CAD build for the part. Positions are in the model's coordinates, mm. A direction names the side the tool comes from. Coordinates: 2 decimals unless noted, no trailing zeros. Order: outer loops, then holes, each group sorted by start corner. A loop starts at its lowest first (then second) coordinate and runs counter-clockwise, first axis right, second up. Notation, with made-up numbers: (5, 16.5) - (41, 16.5) arc R18 ccw to (41, 28.5) - close; hole circle Ø3 at (-21, -3). An arc over 180 degrees is marked (long way). Write each question's results on one line, items separated by ' | '. Start each with the question number.
Q1. Wall check: probe 1 along X at (y, z) = (30.2, 5); probe 2 along Y at (x, z) = (-11, 13.5); probe 3 along Z at (x, y) = (-20.5, 35). Give the ranges that are in metal, low to high.
Q2. Pin check, flat tips, straight feed: P1, Ø4, axis at x = 12, y = 19.5, coming from the -Z side; P2, Ø3, axis at x = -13.75, z = 5, coming from the -Y side; P3, Ø1.5, axis at y = 20, z = -35, coming from the +X side. Stop position of each tip, or through.
Q3. Band-saw the part on C-C, the plane y = 16.5. Write the cut outline in (x, z), then the cut area to 3 significant figures.
Q4. Which spindle directions (+Z, -Z, +X, -X, +Y, -Y) get a long thin tool onto all of the face, cutting with end or side? Do faces 1 (the flat face through (-27, 31.4, -1)), 2 (the flat face through (-27, 29.4, -1)), 3 (the cylindrical face through (52.55, 24.65, -6.9)). Say none if no direction does.
Q5. Band-saw the part on A-A, the plane x = 0. Write the cut outline in (y, z), then the cut area to 3 significant figures.
Q6. Band-saw the part on D-D, the plane x = 12. Write the cut outline in (y, z), then the cut area to 3 significant figures.
Q7. Pull direction X, two halves, no side cores. Call faces 4 (the flat face through (39, 29.4, -1)), 5 (the cylindrical face through (-48.794, 24.65, 25.379)), 6 (the flat face through (39, 31.4, -1)), 7 (the flat face through (29, 0, -45)): released by +X, released by -X, zero draft, split by the parting line, or undercut.
Q8. Band-saw the part on B-B, the plane z = 0. Write the cut outline in (x, y).
```python
from build123d import *

# Parameters (mm, degrees)
SKETCH1_R           = 55
SKETCH1_R_2         = 53
BOSS_EXTRUDE1_DEPTH = 50
RIB7_REACH          = 85.881
SKETCH2_WALL_W      = 256.096361878
SKETCH2_WALL_H      = 2
RIB8_REACH          = 85.881
SKETCH5_WALL_W      = 103.99879807
SKETCH5_WALL_H      = 2
SKETCH6_R           = 1
CUT_EXTRUDE1_DEPTH  = 84.880629468


with BuildPart() as part:
    # Sketch1 → Boss-Extrude1 (new body)
    with BuildSketch(Plane(origin=(0, 0, 0), x_dir=(1, 0, 0), z_dir=(0, 1, 0))):
        with Locations(Location((0, 0, 0), (0, 0, 270))):
            Circle(SKETCH1_R)
        with Locations(Location((0, 0, 0), (0, 0, 270))):
            Circle(SKETCH1_R_2, mode=Mode.SUBTRACT)
    extrude(amount=BOSS_EXTRUDE1_DEPTH)

    # Sketch2 wall → Rib7 (add, up to next)
    with BuildSketch(Plane(origin=(30.75, 31.4, 0), x_dir=(0, 0, 1), z_dir=(1, 0, 0)), mode=Mode.PRIVATE) as rib7_sk1:
        with Locations((0, 1)):
            Rectangle(SKETCH2_WALL_W, SKETCH2_WALL_H)
    rib7_tool1 = extrude(rib7_sk1.sketch, amount=RIB7_REACH, mode=Mode.PRIVATE) - part.part
    add(rib7_tool1.solids().sort_by_distance((30.75, 31.4, 0))[0])

    # Sketch5 wall → Rib8 (add, up to next)
    with BuildSketch(Plane(origin=(-10.25, 31.4, 0), x_dir=(0, 0, 1), z_dir=(1, 0, 0)), mode=Mode.PRIVATE) as rib8_sk1:
        with Locations((0, 1)):
            Rectangle(SKETCH5_WALL_W, SKETCH5_WALL_H)
    rib8_tool1 = extrude(rib8_sk1.sketch, amount=-RIB8_REACH, mode=Mode.PRIVATE) - part.part
    add(rib8_tool1.solids().sort_by_distance((-10.25, 31.4, 0))[0])

    # Sketch6 → Cut-Extrude1 (cut, through all)
    with BuildSketch(Plane(origin=(0, 31.4, 0), x_dir=(1, 0, 0), z_dir=(0, 1, 0))):
        with Locations(Location((-13.75, -5, 0), (0, 0, 270))):
            Circle(SKETCH6_R)
        with Locations(Location((34.25, -5, 0), (0, 0, 270))):
            Circle(SKETCH6_R)
        with Locations(Location((34.25, 5, 0), (0, 0, 270))):
            Circle(SKETCH6_R)
        with Locations(Location((-13.75, 5, 0), (0, 0, 270))):
            Circle(SKETCH6_R)
    extrude(amount=-CUT_EXTRUDE1_DEPTH, mode=Mode.SUBTRACT)


solid = part.part
```
Results below:
1) probe 1: x = -54.77 to -14.75, -12.75 to -10.25, 30.75 to 33.25, 35.25 to 54.77 | probe 2: y = 29.4 to 31.4 | probe 3: z = -51.04 to -48.87, 48.87 to 51.04
2) P1: stops at z = -54.08 | P2: stops at y = 29.4 | P3: stops at x = 43.03
3) outline: circle Ø110 at (0, 0); hole circle Ø106 at (0, 0) | area: 679 mm²
4) face 1: +Y | face 2: -Y | face 3: none
5) outline: (0, -55) - (50, -55) - (50, -53) - (0, -53) - close; (0, 53) - (50, 53) - (50, 55) - (0, 55) - close | area: 200 mm²
6) outline: (0, -53.67) - (50, -53.67) - (50, -51.62) - (0, -51.62) - close; (0, 51.62) - (50, 51.62) - (50, 53.67) - (0, 53.67) - close | area: 205 mm²
7) face 4: undercut | face 5: split by the parting line | face 6: undercut | face 7: zero draft
8) outline: (-55, 0) - (-53, 0) - (-53, 29.4) - (-10.25, 29.4) - (-10.25, 31.4) - (-53, 31.4) - (-53, 50) - (-55, 50) - close; (30.75, 29.4) - (53, 29.4) - (53, 0) - (55, 0) - (55, 50) - (53, 50) - (53, 31.4) - (30.75, 31.4) - close
